Build history of the part. All positions in model axes, mm. Give positions to 0.01 mm unless a question says otherwise; leave off trailing zeros. Loops run counter-clockwise (first coordinate to the right, second up) from the corner with the lowest first, then second, coordinate; pieces in that order, holes last. Notation, with made-up numbers: (-40, 16) -> (-10, 16) arc R35 ccw to (-10, 50) -> close; hole circle Ø9 at (-32, -14). An arc over 180 degrees is marked (long way). Answer in a Markdown table with one row per item. Add a question column.
from build123d import *

# Parameters (mm, degrees)
EXTRUDE_2_DEPTH     = 10
SKETCH_2_R          = 10
CUT_EXTRUDE_2_DEPTH = 10


with BuildPart() as part:
    # Эскиз1 → Бобышка-Вытянуть2 (new body)
    with BuildSketch(Plane.XY):
        with BuildLine():
            Line((0, 25), (200, 25))
            ThreePointArc((200, 25), (225, 0), (200, -25))
            Line((200, -25), (0, -25))
            ThreePointArc((0, -25), (-25, 0), (0, 25))
        make_face()
    extrude(amount=EXTRUDE_2_DEPTH)

    # Эскиз2 → Вырез-Вытянуть2 (cut)
    with BuildSketch(Plane.XY.offset(10)):
        Circle(SKETCH_2_R)
        with Locations((200, 0)):
            Circle(SKETCH_2_R)
    extrude(amount=-CUT_EXTRUDE_2_DEPTH, mode=Mode.SUBTRACT)


solid = part.part
(1) Flat gauge pin, fed straight in: pin 1 Ø3 at (x, y) = (173, 11) entering from -Z. Where does the tip first touch, or does it go through?
(2) Two-plate mould, pull along X, no slides. Class faces 1 (the cylindrical face through (209.237, -3.83, 5.07)), 2 (the flat face through (101, -25, 5)), 3 (the cylindrical face through (-24.994, -0.55, 4.93)): released by +X, released by -X, zero draft, split by the parting line, or undercut.
(3) Saw through at C-C, the plane x = 195. List the corners of the cut face in (y, z), then the cut area to 3 significant figures.
(4) Saw through at B-B, the plane z = 4.25. List the corners of the cut face in (x, y), then the cut area to 3 significant figures.
(5) Saw through at A-A, the plane y = 0. List the corners of the cut face in (x, z), then the cut area to 3 significant figures.
(6) Wall check: line 1 along X through (y, z) = (-1, 9.5); line 2 along X through (y, z) = (0.5, 8.5) (1 decimal); line 3 along Y through (x, z) = (0, 3.5). Give the ranges that are in metal, low to high. Write a range as from..to.
Worked answers:
| question | item | result |
|---|---|---|
| 1 | pin 1 | z = 0 |
| 2 | face 1 | undercut |
| 2 | face 2 | zero draft |
| 2 | face 3 | released by -X |
| 3 | outline | (-25, 0) -> (-8.66, 0) -> (-8.66, 10) -> (-25, 10) -> close; (8.66, 0) -> (25, 0) -> (25, 10) -> (8.66, 10) -> close |
| 3 | area | 327 mm^2 |
| 4 | outline | (0, -25) -> (200, -25) arc R25 ccw to (200, 25) -> (0, 25) arc R25 ccw to start; hole circle Ø20 at (0, 0); hole circle Ø20 at (200, 0) |
| 4 | area | 11,300 mm^2 |
| 5 | outline | (-25, 0) -> (-10, 0) -> (-10, 10) -> (-25, 10) -> close; (10, 0) -> (190, 0) -> (190, 10) -> (10, 10) -> close; (210, 0) -> (225, 0) -> (225, 10) -> (210, 10) -> close |
| 5 | area | 2,100 mm^2 |
| 6 | line 1 | -24.98..-9.95, 9.95..190.05, 209.95..224.98 |
| 6 | line 2 | -25..-10, 10..190, 210..225 |
| 6 | line 3 | -25..-10, 10..25 |
